Geometry check sheet. Reference: the model listing, model coordinates, mm. Face numbers are marked on the shaded views. A direction names the side the tool comes from. Give positions to 0.01 mm unless a question says otherwise; leave off trailing zeros. Loops run counter-clockwise (first coordinate to the right, second up) from the corner with the lowest first, then second, coordinate; pieces in that order, holes last. Notation, with made-up numbers: (13, -18.75) - (31, -18.75) arc R21 ccw to (31, -9.75) - close; hole circle Ø3 at (-36, 88). An arc over 180 degrees is marked (long way). One line per question, with ' | ' between items. Start each with the question number.
Autodesk Inventor part; units mm, degrees
ref_plane "工作平面2" through (-212.499, 20.5, 0) normal (-1, 0, 0) x (0, 0, 1)
ref_plane "YZ Plane" through (0, 0, 0) normal (1, 0, 0) x (0, 1, 0)
ref_plane "XZ Plane" through (0, 0, 0) normal (0, 1, 0) x (-1, 0, 0)
sketch "草图1" plane through (0, 0, 0) normal (0, 1, 0) x (-1, 0, 0)
  circle A0 centre (0, 0) radius 5
  dimension "d0" = 10
extrude "拉伸1" add sketch "草图1" along normal blind 2
sketch "草图2" plane through (0, 2, 0) normal (0, 1, 0) x (1, 0, 0)
  circle A0 centre (0, 0) radius 5
  circle A1 centre (0, 0) radius 4
  dimension "d3" = 8
extrude "拉伸2" add sketch "草图2" along normal blind 1 contours A1
sketch "草图3" plane through (0, 3, 0) normal (0, 1, 0) x (1, 0, 0)
  circle A0 centre (0, 0) radius 5
extrude "拉伸3" add sketch "草图3" along normal blind 5
sketch "草图4" plane through (0, 0, 0) normal (0, -1, 0) x (1, 0, 0)
  circle A0 centre (0, 0) radius 5
  circle A1 centre (0, 0) radius 4
extrude "拉伸4" add sketch "草图4" along normal blind 1
sketch "草图5" plane through (0, 8, 0) normal (0, 1, 0) x (1, 0, 0)
  circle A0 centre (0, 0) radius 6
  dimension "d10" = 12
extrude "拉伸5" add sketch "草图5" along normal blind 5
sketch "草图6" plane through (0, 13, 0) normal (0, 1, 0) x (1, 0, 0)
  line L0 (-10, -10) -> (10, -10)
  line L1 (10, -10) -> (10, 10)
  line L2 (10, 10) -> (-10, 10)
  line L3 (-10, 10) -> (-10, -10)
  line L4 (-10, -10) -> (10, 10) construction
  line L5 (10, -10) -> (-10, 10) construction
  point P0 (0, 0)
  dimension "d13" = 20
extrude "拉伸6" add sketch "草图6" along normal blind 15
sketch "草图7" plane through (-10, 13, -10) normal (-1, 0, 0) x (0, 0, 1)
  line L0 (20, 0) -> (20, 15) construction
  line L1 (20, 0) -> (0, 0) construction
  line L2 (20, 15) -> (0, 0) construction
  line L3 (20, 0) -> (0, 15) construction
  circle A0 centre (10, 7.5) radius 3.5
  point P0 (10, -13)
  dimension "d16" = 7
extrude "拉伸7" add sketch "草图7" along normal blind 150
sketch "草图8" plane through (-160, 20.5, 0) normal (-1, 0, 0) x (0, 0, 1)
  line L0 (-4.7374, 5.2626) -> (5.2626, 5.2626)
  line L1 (5.2626, 5.2626) -> (5.2626, -4.7374)
  line L2 (5.2626, -4.7374) -> (-4.7374, -4.7374)
  line L3 (-4.7374, -4.7374) -> (-4.7374, 5.2626)
  line L4 (-4.7374, 5.2626) -> (5.2626, -4.7374) construction
  line L5 (5.2626, 5.2626) -> (-4.7374, -4.7374) construction
  point P0 (0, -20.5)
  point P1 (0.2626, 0.2626)
  dimension "d19" = 10
extrude "拉伸8" add sketch "草图8" along normal blind 2
sketch "草图9" plane through (-162, 20.5, 0) normal (-1, 0, 0) x (0, 0, 1)
  line L0 (0, 0) -> (0, 3) construction
  line L1 (0, 0) -> (-2.5981, -1.5) construction
  line L2 (0, 0) -> (2.5981, -1.5) construction
  line L3 (0, 0) -> (-4.7226, 0) construction
  circle A0 centre (-2.5981, 1.5) radius 2
  circle A1 centre (0, -3) radius 2
  circle A2 centre (2.5981, 1.5) radius 2
  point P0 (0, -20.5)
  dimension "d22" = 120
  dimension "d23" = 120
  dimension "d24" = 3
  dimension "d26" = 3
  dimension "d27" = 3
ref_plane "工作平面2" through (-212.499, 20.5, 0) normal (-1, 0, 0) x (0, 0, 1)
ref_plane "工作平面1" through (-161, 20.5, 0) normal (-1, 0, 0) x (0, 0, 1)
sketch "草图10" plane through (-212.499, 20.5, 0) normal (-1, 0, 0) x (0, 0, 1)
  line L0 (0, 18.3) -> (0, -29.3) construction
  line L1 (-30.8, -20.5) -> (30.8, -20.5) construction
  circle A0 centre (0, -20.5) radius 2
  circle A1 centre (-20, 9.5) radius 2
  circle A2 centre (20, 9.5) radius 2
  dimension "d32" = 4
  dimension "d33" = 4
  dimension "d34" = 30
  dimension "d35" = 20
loft "放样1" add profiles "草图10", "草图9" contours A0 / A1
loft "放样2" add profiles "草图9", "草图10" contours A2 / A2
loft "放样3" add profiles "草图9", "草图10" contours A0 / A1
properties part number "摄像头" material "橡胶"
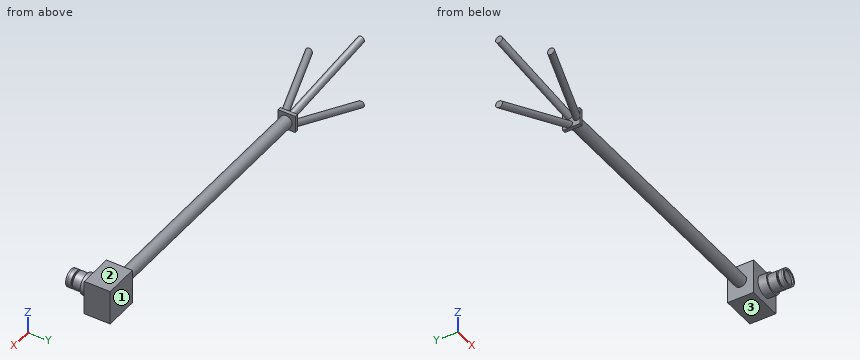
(1) Section check B-B, the plane x = -130. Record the boundary of the cut face in (y, z).
(2) Tool access check on the marked faces 1, 2 and 3. Record the directions out of +Z, -Z, +X, -X, +Y, -Y that give a thin tool (end or side, any length) a straight path to the whole face; none if there is none.
(3) Material ranges on line 1 (Z direction, x = 0, y = -0.7); line 2 (Z direction, x = -8, y = 14), recorded low to high.
(4) Depth check by flat-ended pin: pin 1 Ø12 at (x, y) = (-3.5, 21.5) entering from -Z; pin 2 Ø1.5 at (y, z) = (2.5, -1.5) entering from +X; pin 3 Ø6 at (x, y) = (-26.5, 24.5) entering from +Z; pin 4 Ø5 at (x, y) = (-34.5, 13.5) entering from +Z. Enter the tip coordinate at first touch or a pass-through.
(5) Section check A-A, the plane x = 0. Record the boundary of the cut face in (y, z).
Numbers:
1) outline: circle Ø7 at (20.5, 0)
2) face 1: +Z, -Z, +X, -X, +Y | face 2: +Z, +X, +Y, -Y | face 3: -Z, +X, +Y, -Y
3) line 1: -5 to -4, 4 to 5 | line 2: -10 to 10
4) pin 1: z = -10 | pin 2: x = 4.91 | pin 3: z = 3.35 | pin 4: through
5) outline: (-1, -5) - (2, -5) - (2, -4) - (3, -4) - (3, -5) - (8, -5) - (8, -6) - (13, -6) - (13, -10) - (28, -10) - (28, 10) - (13, 10) - (13, 6) - (8, 6) - (8, 5) - (3, 5) - (3, 4) - (2, 4) - (2, 5) - (-1, 5) - (-1, 4) - (0, 4) - (0, -4) - (-1, -4) - close
